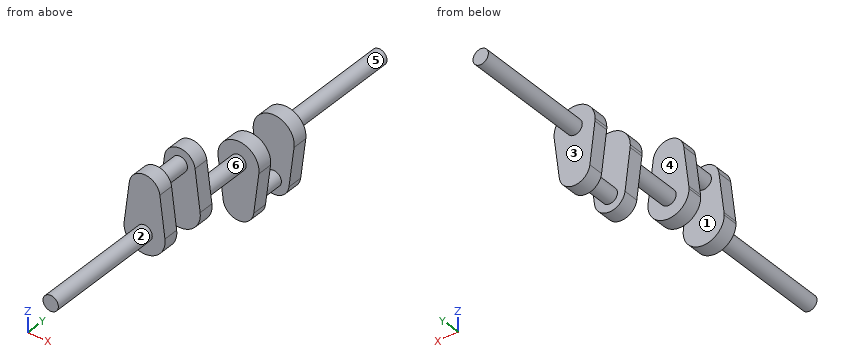
```python
from build123d import *

# Parameters (mm, degrees)
F0_R      = 9.525
F1_DEPTH  = 152.4
F2_R      = 9.525
F3_DEPTH  = 19.05
F4_R      = 9.525
F5_DEPTH  = 38.1
F7_DEPTH  = 19.05
F8_R      = 9.525
F9_DEPTH  = 76.2
F11_DEPTH = 19.05
F12_R     = 9.525
F13_DEPTH = 38.1
F15_DEPTH = 19.05
F16_R     = 9.525
F17_DEPTH = 152.4


with BuildPart() as f1:
    # F0 (on Front) → F1 (new body)
    with BuildSketch(Plane.XZ):
        Circle(F0_R)
    extrude(amount=F1_DEPTH)

    # F2 (on face) → F3 (join)
    with BuildSketch(Plane(origin=(0, 0, 0), x_dir=(-1, 0, 0), z_dir=(0, 1, 0))):
        with BuildLine():
            ThreePointArc((-18.9005859708, 53.1812496635), (-1.1929663147, 31.7873902009), (19.05, 50.8))
            ThreePointArc((19.05, 50.8), (19.012609793, 51.992966411), (18.9005859467, 53.1812498549))
            ThreePointArc((18.9005859467, 53.1812498549), (-9.64e-08, 69.85), (-18.9005859708, 53.1812496635))
        make_face()
        with Locations((0, 50.8)):
            Circle(F2_R, mode=Mode.SUBTRACT)
        with BuildLine():
            ThreePointArc((18.9005859467, 53.1812498549), (19.012609793, 51.992966411), (19.05, 50.8))
            ThreePointArc((19.05, 50.8), (-1.1929663147, 31.7873902009), (-18.9005859708, 53.1812496635))
            Line((-18.9005859708, 53.1812496635), (-25.2007812071, 3.1750002442))
            ThreePointArc((-25.2007812071, 3.1750002442), (2.614e-07, 25.4), (25.2007812725, 3.1749997256))
            Line((25.2007812725, 3.1749997256), (18.9005859467, 53.1812498549))
        make_face()
        with BuildLine():
            ThreePointArc((25.4, 0), (25.3501463933, 1.5906218406), (25.2007812725, 3.1749997256))
            ThreePointArc((25.2007812725, 3.1749997256), (2.614e-07, 25.4), (-25.2007812071, 3.1750002442))
            ThreePointArc((-25.2007812071, 3.1750002442), (-1.5906221014, -25.3501463769), (25.4, 0))
        make_face()
        with Locations((0, 50.8)):
            Circle(F2_R)
    extrude(amount=F3_DEPTH)

    # F4 (on face) → F5 (join)
    with BuildSketch(Plane(origin=(0, 19.05, 0), x_dir=(-1, 0, 0), z_dir=(0, 1, 0))):
        with Locations((0, 50.8)):
            Circle(F4_R)
    extrude(amount=F5_DEPTH)

    # F6 (on face) → F7 (join)
    with BuildSketch(Plane(origin=(0, 57.15, 0), x_dir=(-1, 0, 0), z_dir=(0, 1, 0))):
        with BuildLine():
            ThreePointArc((-18.9005859708, 53.1812496635), (-1.1929663147, 31.7873902009), (19.05, 50.8))
            ThreePointArc((19.05, 50.8), (19.0126097893, 51.9929664704), (18.9005859318, 53.1812499732))
            ThreePointArc((18.9005859318, 53.1812499732), (-1.561e-07, 69.85), (-18.9005859708, 53.1812496635))
        make_face()
        with BuildLine():
            ThreePointArc((18.9005859318, 53.1812499732), (19.0126097893, 51.9929664704), (19.05, 50.8))
            ThreePointArc((19.05, 50.8), (-1.1929663147, 31.7873902009), (-18.9005859708, 53.1812496635))
            Line((-18.9005859708, 53.1812496635), (-25.200781271, 3.1749997374))
            ThreePointArc((-25.200781271, 3.1749997374), (-1.19e-07, 25.4), (25.2007812412, 3.1749999736))
            Line((25.2007812412, 3.1749999736), (18.9005859318, 53.1812499732))
        make_face()
        with BuildLine():
            ThreePointArc((25.4, 0), (25.3501463854, 1.5906219653), (25.2007812412, 3.1749999736))
            ThreePointArc((25.2007812412, 3.1749999736), (-1.19e-07, 25.4), (-25.200781271, 3.1749997374))
            ThreePointArc((-25.200781271, 3.1749997374), (-1.5906218465, -25.3501463929), (25.4, 0))
        make_face()
    extrude(amount=F7_DEPTH)

    # F8 (on face) → F9 (join)
    with BuildSketch(Plane(origin=(0, 76.2, 0), x_dir=(-1, 0, 0), z_dir=(0, 1, 0))):
        Circle(F8_R)
    extrude(amount=F9_DEPTH)

    # F10 (on face) → F11 (join)
    with BuildSketch(Plane(origin=(0, 152.4, 0), x_dir=(-1, 0, 0), z_dir=(0, 1, 0))):
        with BuildLine():
            ThreePointArc((25.2007812725, -3.1749997255), (25.3501463933, -1.5906218405), (25.4, 0))
            ThreePointArc((25.4, 0), (-1.5906219941, 25.3501463836), (-25.200781234, -3.1750000308))
            ThreePointArc((-25.200781234, -3.1750000308), (1.539e-07, -25.4), (25.2007812725, -3.1749997255))
        make_face()
        with BuildLine():
            ThreePointArc((25.2007812725, -3.1749997255), (1.539e-07, -25.4), (-25.200781234, -3.1750000308))
            Line((-25.200781234, -3.1750000308), (-18.9005859708, -53.1812496635))
            ThreePointArc((-18.9005859708, -53.1812496635), (-1.1929663147, -31.7873902009), (19.05, -50.8))
            ThreePointArc((19.05, -50.8), (19.012609782, -51.9929665866), (18.9005859027, -53.1812502041))
            Line((18.9005859027, -53.1812502041), (25.2007812725, -3.1749997255))
        make_face()
        with BuildLine():
            ThreePointArc((19.05, -50.8), (-1.1929663147, -31.7873902009), (-18.9005859708, -53.1812496635))
            ThreePointArc((-18.9005859708, -53.1812496635), (-2.724e-07, -69.85), (18.9005859027, -53.1812502041))
            ThreePointArc((18.9005859027, -53.1812502041), (19.012609782, -51.9929665866), (19.05, -50.8))
        make_face()
    extrude(amount=F11_DEPTH)

    # F12 (on face) → F13 (join)
    with BuildSketch(Plane(origin=(0, 171.45, 0), x_dir=(-1, 0, 0), z_dir=(0, 1, 0))):
        with Locations((0, -50.8)):
            Circle(F12_R)
    extrude(amount=F13_DEPTH)

    # F14 (on face) → F15 (join)
    with BuildSketch(Plane(origin=(0, 209.55, 0), x_dir=(-1, 0, 0), z_dir=(0, 1, 0))):
        with BuildLine():
            ThreePointArc((18.900585933, -53.1812499633), (19.0126097896, -51.9929664655), (19.05, -50.8))
            ThreePointArc((19.05, -50.8), (-1.1929664809, -31.7873902114), (-18.9005859292, -53.1812499939))
            ThreePointArc((-18.9005859292, -53.1812499939), (1.54e-08, -69.85), (18.900585933, -53.1812499633))
        make_face()
        with BuildLine():
            ThreePointArc((-18.9005859292, -53.1812499939), (-1.1929664809, -31.7873902114), (19.05, -50.8))
            ThreePointArc((19.05, -50.8), (19.0126097896, -51.9929664655), (18.900585933, -53.1812499633))
            Line((18.900585933, -53.1812499633), (25.2007812062, -3.1750002518))
            ThreePointArc((25.2007812062, -3.1750002518), (2.227e-07, -25.4), (-25.2007811505, -3.1750006937))
            Line((-25.2007811505, -3.1750006937), (-18.9005859292, -53.1812499939))
        make_face()
        with BuildLine():
            ThreePointArc((25.4, 0), (-1.5906223275, 25.3501463627), (-25.2007811505, -3.1750006937))
            ThreePointArc((-25.2007811505, -3.1750006937), (2.227e-07, -25.4), (25.2007812062, -3.1750002518))
            ThreePointArc((25.2007812062, -3.1750002518), (25.3501463767, -1.5906221053), (25.4, 0))
        make_face()
    extrude(amount=F15_DEPTH)

    # F16 (on face) → F17 (join)
    with BuildSketch(Plane(origin=(0, 228.6, 0), x_dir=(-1, 0, 0), z_dir=(0, 1, 0))):
        Circle(F16_R)
    extrude(amount=F17_DEPTH)


solid = f1.part
```
CAD build for the part. Positions are in the model's coordinates, mm. Face numbers are marked on the shaded views. A direction names the side the tool comes from. Round coordinates to 2 decimals unless told otherwise and drop trailing zeros. Write each loop counter-clockwise with the first axis right and the second up, starting at its lowest first coordinate (ties: lowest second). Pieces come first, ordered by that corner, then holes. Notation, with made-up numbers: (83, 15) - (107, 15) arc R21 ccw to (107, 42) - close; hole circle Ø4 at (44, 80.5). An arc over 180 degrees is marked (long way). Write item = value, one per line. Start each with the question number.
Q1. Probe L1, parallel to Y at x = -13.5, z = 2; L2, parallel to Y at x = 12.5, z = -64; L3, parallel to Y at x = 16.5, z = 44.5. List the from-to ranges inside material, lowest first. Write a range as from..to.
Q2. Drop flat-ended pins along their axis: pin 1 (15 mm diameter, centred on x = 12, z = -39, fed in from -Y); pin 2 (15 mm diameter, centred on x = -1.5, z = 44, fed in from -Y); pin 3 (8 mm diameter, centred on x = 1, y = 322.5, fed in from +Z) (3 decimals). Give the stop position or say it passes through.
Q3. Band-saw the part on A-A (z = -16.5). Give the cut face in (x, y).
Q4. Band-saw the part on C-C (y = 220.5). Give the cut face in (x, z) (3 decimals).
Q5. Which spindle directions (+Z, -Z, +X, -X, +Y, -Y) get a long thin tool onto all of the face, cutting with end or side? Do the marked faces 5 and 6. Say none if no direction does.
Q6. Mould opens along Y. For the marked faces 1, 2, 3 and 4 say: pulls with the +Y half, pulls with the -Y half, needs draft (parallel to the pull), parting line crosses it, or undercut.
Q7. Band-saw the part on B-B (z = 31.5). Give the cut face in (x, y), then the cut area to 3 significant figures.
Answers below:
q1.L1 = 0..19.05, 57.15..76.2, 152.4..171.45, 209.55..228.6
q1.L2 = 152.4..171.45, 209.55..228.6
q1.L3 = 0..19.05, 57.15..76.2
q2.pin_1 = 152.4
q2.pin_2 = 0
q2.pin_3 = 9.525
q3.outline = (-23.52, 152.4) - (23.52, 152.4) - (23.52, 171.45) - (-23.52, 171.45) - close; (-23.52, 209.55) - (23.52, 209.55) - (23.52, 228.6) - (-23.52, 228.6) - close; (-19.31, 0) - (19.31, 0) - (19.31, 19.05) - (-19.31, 19.05) - close; (-19.31, 57.15) - (19.31, 57.15) - (19.31, 76.2) - (-19.31, 76.2) - close
q4.outline = (-25.201, -3.175) - (-18.901, -53.181) arc R19.05 ccw to (18.901, -53.181) - (25.201, -3.175) arc R25.4 ccw (long way) to start
q5.face_5 = +Y
q5.face_6 = none
q6.face_1 = undercut
q6.face_2 = needs draft
q6.face_3 = pulls with the +Y half
q6.face_4 = undercut
q7.outline = (-21.63, 0) - (21.63, 0) - (21.63, 19.05) - (-21.63, 19.05) - close; (-21.63, 57.15) - (21.63, 57.15) - (21.63, 76.2) - (-21.63, 76.2) - close
q7.area = 1,650 mm2
